from build123d import *

# Parameters (mm, degrees)
F1_DEPTH = 30
F2_R     = 4.4
F3_R     = 4.4
F4_DEPTH = 25
F5_R     = 2
F6_R     = 2


# Not quite as in the source:
# - a feature names something its author has since deleted; it is built from what else it names


with BuildPart() as f1:
    # F0 (on Front) → F1 (new body)
    with BuildSketch(Plane.XZ):
        Polygon((90, -1), (90, 1), (70, 1), (70, 89), (-70, 89), (-70, 1), (-90, 1), (-90, -1), (-68, -1), (-68, 87), (68, 87), (68, -1), align=None)
    extrude(amount=F1_DEPTH)

    # F2 (on face) + F3 (on face) → F4 (cut)
    with BuildSketch(Plane.XY.offset(1)):
        with Locations((-80, -15)):
            Circle(F2_R)
        with Locations((80, -15)):
            Circle(F2_R)
    with BuildSketch(Plane.XY.offset(89)):
        with Locations((-25, -15)):
            Circle(F3_R)
        with Locations((25, -15)):
            Circle(F3_R)
    extrude(amount=-F4_DEPTH, mode=Mode.SUBTRACT)

    # F5
    f5_edges = [f1.edges().sort_by_distance(p)[0] for p in [
        (-70, -15, 89),
        (70, -15, 89),
    ]]
    fillet(f5_edges, radius=F5_R)

    # F6
    f6_edges = [f1.edges().sort_by_distance(p)[0] for p in [
        (68, -15, -1),
        (-68, -15, -1),
    ]]
    fillet(f6_edges, radius=F6_R)


solid = f1.part
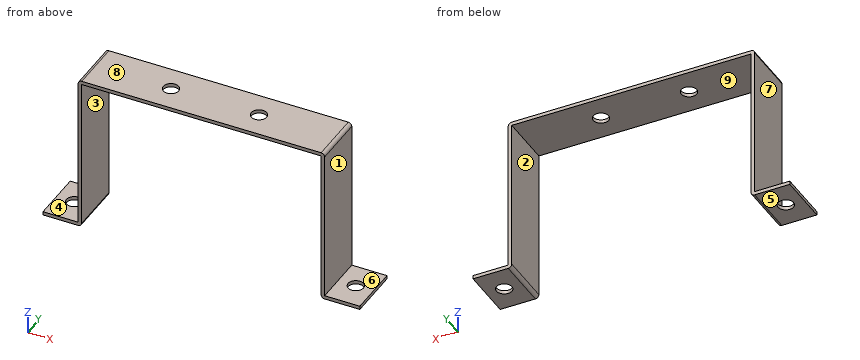
The model under review builds one solid part; all positions refer to its coordinate system, in mm. Face numbers are marked on the shaded views. A direction names the side the tool comes from. Coordinates: 2 decimals unless noted, no trailing zeros. Write each loop counter-clockwise with the first axis right and the second up, starting at its lowest first coordinate (ties: lowest second). Pieces come first, ordered by that corner, then holes. Notation, with made-up numbers: (-34, 42) -> (13, 42) arc R15 cw to (13, 63) -> close; hole circle Ø2 at (22.25, 63). An arc over 180 degrees is marked (long way). Answer in a Markdown table with one row per item.
1. For the marked faces 5, 6, 7, 8 and 9, list the 3-axis set-ups (+Z, -Z, +X, -X, +Y, -Y) from which the entire face can be reached by the end or side of a thin tool; tool diameter is ignored.
Answers below:
| item | result |
|---|---|
| face 5 | -Z, +X, -X, +Y, -Y |
| face 6 | +Z, +X, +Y, -Y |
| face 7 | +Z, -X, +Y, -Y |
| face 8 | +Z, +X, -X, +Y, -Y |
| face 9 | -Z, +Y, -Y |
2. We need section D-D, the plane y = -23. State the section outline as (x, z) points.
Answers below:
| item | result |
|---|---|
| outline | (-90, -1) -> (-70, -1) arc R2 ccw to (-68, 1) -> (-68, 87) -> (68, 87) -> (68, 1) arc R2 ccw to (70, -1) -> (90, -1) -> (90, 1) -> (70, 1) -> (70, 87) arc R2 ccw to (68, 89) -> (-68, 89) arc R2 ccw to (-70, 87) -> (-70, 1) -> (-90, 1) -> close |
3. Wall thickness on probe 1 along X at (y, z) = (-28, 9.5); probe 2 along Y at (x, z) = (-80, 0.35); probe 3 along Z at (x, y) = (-12, -15.5): over which ranges is each line inside the solid? List them lowest first. Write a range as [from, to].
Answers below:
| item | result |
|---|---|
| probe 1 | x = [-70, -68], [68, 70] |
| probe 2 | y = [-30, -19.4], [-10.6, 0] |
| probe 3 | z = [87, 89] |
4. Clearance check with flat-ended pins moving along their axes: pin 1 Ø1.5 at (x, y) = (61.5, -12.5) entering from -Z; pin 2 Ø2 at (x, y) = (70, -9) entering from +Z; pin 3 Ø1 at (y, z) = (-3.5, 70.5) entering from +X; pin 4 Ø5.5 at (x, y) = (-80, -15) entering from -Z. State where each tip first meets the part, or that it passes through.
Answers below:
| item | result |
|---|---|
| pin 1 | stops at z = 87 |
| pin 2 | stops at z = 88.73 |
| pin 3 | stops at x = 70 |
| pin 4 | passes through |
5. We need section C-C, the plane y = -15. Give the number of separate pieces and of enclosed holes in the cut face, and give its area (3 significant figures).
Answers below:
| item | result |
|---|---|
| separate pieces | 5 |
| enclosed holes | 0 |
| area | 638 mm^2 |
6. We need section A-A, the plane x = 80. State the section outline as (y, z) points.
Answers below:
| item | result |
|---|---|
| outline | (-30, -1) -> (-19.4, -1) -> (-19.4, 1) -> (-30, 1) -> close; (-10.6, -1) -> (0, -1) -> (0, 1) -> (-10.6, 1) -> close |
7. We need section B-B, the plane z = 41. State the section outline as (x, y) points.
Answers below:
| item | result |
|---|---|
| outline | (-70, -30) -> (-68, -30) -> (-68, 0) -> (-70, 0) -> close; (68, -30) -> (70, -30) -> (70, 0) -> (68, 0) -> close |
8. Draft analysis for pull direction X (two halves, no side actions). For the marked faces 1, 2, 3 and 4, state which applies: +X half, -X half, draft (parallel to the pull), parting line (faces both ways), or undercut.
Answers below:
| item | result |
|---|---|
| face 1 | +X half |
| face 2 | undercut |
| face 3 | undercut |
| face 4 | draft |
